from build123d import *

# Parameters (mm, degrees)
SKETCH1_R           = 10.95
SKETCH1_R_2         = 9.5
BOSS_EXTRUDE1_DEPTH = 0.8
SKETCH2_W           = 2
SKETCH2_H           = 14.789010462
CUT_EXTRUDE1_DEPTH  = 16.506289047
SKETCH3_W           = 2.5
SKETCH3_H           = 2.5
BOSS_EXTRUDE2_DEPTH = 0.8
FILLET1_R           = 0.5
FILLET2_R           = 0.5
SKETCH4_R           = 0.85
CUT_EXTRUDE2_DEPTH  = 16.506289047


with BuildPart() as part:
    # Sketch1 → Boss-Extrude1 (new body)
    with BuildSketch(Plane.XY):
        Circle(SKETCH1_R)
        Circle(SKETCH1_R_2, mode=Mode.SUBTRACT)
    extrude(amount=BOSS_EXTRUDE1_DEPTH)

    # Sketch2 → Cut-Extrude1 (cut, through all)
    with BuildSketch(Plane.XY.offset(0.8)):
        with Locations((0, 7.394505231)):
            Rectangle(SKETCH2_W, SKETCH2_H)
    extrude(amount=-CUT_EXTRUDE1_DEPTH, mode=Mode.SUBTRACT)

    # Sketch3 → Boss-Extrude2 (add)
    with BuildSketch(Plane.XY.offset(0.8)):
        with Locations((2.25, 8.197221814)):
            Rectangle(SKETCH3_W, SKETCH3_H)
        with Locations((-2.25, 8.197221814)):
            Rectangle(SKETCH3_W, SKETCH3_H)
    extrude(amount=-BOSS_EXTRUDE2_DEPTH)

    # Fillet1
    fillet1_edges = [part.edges().sort_by_distance(p)[0] for p in [
        (1, 10.904242294, 0.4),
        (-1, 10.904242294, 0.4),
        (3.5, 8.831760866, 0.4),
        (-3.5, 8.831760866, 0.4),
    ]]
    fillet(fillet1_edges, radius=FILLET1_R)

    # Fillet2
    fillet2_edges = [part.edges().sort_by_distance(p)[0] for p in [
        (1, 6.947221814, 0.4),
        (3.5, 6.947221814, 0.4),
        (-1, 6.947221814, 0.4),
        (-3.5, 6.947221814, 0.4),
    ]]
    fillet(fillet2_edges, radius=FILLET2_R)

    # Sketch4 → Cut-Extrude2 (cut, through all)
    with BuildSketch(Plane.XY.offset(0.8)):
        with Locations((2.25, 8.447221814)):
            Circle(SKETCH4_R)
        with Locations((-2.25, 8.447221814)):
            Circle(SKETCH4_R)
    extrude(amount=-CUT_EXTRUDE2_DEPTH, mode=Mode.SUBTRACT)


solid = part.part
Geometry check sheet. Reference: the model listing, model coordinates, mm. Round coordinates to 2 decimals unless told otherwise and drop trailing zeros. Order: outer loops, then holes, each group sorted by start corner. A loop starts at its lowest first (then second) coordinate and runs counter-clockwise, first axis right, second up. Notation, with made-up numbers: (26, 43) -> (39, 43) arc R12 ccw to (39, 62) -> close; hole circle Ø5 at (34, 87). An arc over 180 degrees is marked (long way). Use one line per item in the form item = value.
1. Cross-section at B-B, the plane x = 2.25. Enter the section's corners in (y, z), plus the area to 3 significant figures.
Working result:
outline = (-10.72, 0) -> (-9.23, 0) -> (-9.23, 0.8) -> (-10.72, 0.8) -> close; (6.95, 0) -> (7.6, 0) -> (7.6, 0.8) -> (6.95, 0.8) -> close; (9.3, 0) -> (10.72, 0) -> (10.72, 0.8) -> (9.3, 0.8) -> close
area = 2.84 mm^2
2. Mould release check, pull along X, two halves, no side actions. Record for faces 1 (the face through (-0.46, -10.94, 0.39)), 2 (the face through (3.06, 8.7, 0.41)), 3 (the face through (-1.7, 7.3, 0)): pulls with the +X half, pulls with the -X half, needs draft (parallel to the pull), parting line crosses it, or undercut.
Working result:
face_1 = parting line crosses it
face_2 = undercut
face_3 = needs draft
3. Cross-section at A-A, the plane y = 0. Enter the section's corners in (x, z).
Working result:
outline = (-10.95, 0) -> (-9.5, 0) -> (-9.5, 0.8) -> (-10.95, 0.8) -> close; (9.5, 0) -> (10.95, 0) -> (10.95, 0.8) -> (9.5, 0.8) -> close
4. Cross-section at C-C, the plane y = 9. Enter the section's corners in (x, z), plus the area to 3 significant figures.
Working result:
outline = (-6.24, 0) -> (-2.9, 0) -> (-2.9, 0.8) -> (-6.24, 0.8) -> close; (-1.6, 0) -> (-1, 0) -> (-1, 0.8) -> (-1.6, 0.8) -> close; (1, 0) -> (1.6, 0) -> (1.6, 0.8) -> (1, 0.8) -> close; (2.9, 0) -> (6.24, 0) -> (6.24, 0.8) -> (2.9, 0.8) -> close
area = 6.31 mm^2
5. Cross-section at D-D, the plane z = 0.25. Enter the section's corners in (x, y), plus the area to 3 significant figures.
Working result:
outline = (-4.22, 8.51) arc R0.5 cw to (-3.5, 8.06) -> (-3.5, 7.45) arc R0.5 ccw to (-3, 6.95) -> (-1.5, 6.95) arc R0.5 ccw to (-1, 7.45) -> (-1, 10.34) arc R0.5 ccw to (-1.57, 10.84) arc R10.95 ccw (long way) to (1.57, 10.84) arc R0.5 ccw to (1, 10.34) -> (1, 7.45) arc R0.5 ccw to (1.5, 6.95) -> (3, 6.95) arc R0.5 ccw to (3.5, 7.45) -> (3.5, 8.06) arc R0.5 cw to (4.22, 8.51) arc R9.5 cw (long way) to start; hole circle Ø1.7 at (-2.25, 8.45); hole circle Ø1.7 at (2.25, 8.45)
area = 96.9 mm^2
6. Scan lines: line 1 along Y through (x, z) = (-2.25, 0.2); line 2 along X through (y, z) = (0, 0.3); line 3 along X through (y, z) = (7.25, 0.35). Record each from-to range of solid material in increasing order. Write a range as from..to.
Working result:
line_1 = -10.72..-9.23, 6.95..7.6, 9.3..10.72
line_2 = -10.95..-9.5, 9.5..10.95
line_3 = -8.21..-6.14, -3.46..-1.04, 1.04..3.46, 6.14..8.21
7. Go/stop test with a flat-tipped pin: pin 1 (11.5 mm diameter, centred on x = 0, y = 0, fed in from -Z). Record where the tip stops, or that it passes through.
Working result:
pin_1 = through
